Verification items for the finished model (mm, model axes). A direction names the side the tool comes from. Give positions to 0.01 mm unless a question says otherwise; leave off trailing zeros. Order: outer loops, then holes, each group sorted by start corner. A loop starts at its lowest first (then second) coordinate and runs counter-clockwise, first axis right, second up. Notation, with made-up numbers: (12, 57.25) -> (33, 57.25) arc R19 ccw to (33, 64.25) -> close; hole circle Ø10 at (88.5, -39). An arc over 180 degrees is marked (long way). Return JSON: item names as keys, results as strings. Group by question number.
(1) Release check for a two-part mould opening along Y. For faces 1 (the face through (-17.056, 75.535, 11.827)), 2 (the face through (0, 5, 28)), 3 (the face through (16.944, 75.535, 11.827)), 4 (the face through (17.06, 41.09, 31.03)) record: pulls with the +Y half, pulls with the -Y half, needs draft (parallel to the pull), parting line crosses it, or undercut.
(2) Thickness scan on line 1 along X through (y, z) = (2.75, 20); line 2 along X through (y, z) = (11, 5.5); line 3 along X through (y, z) = (3, 10). Record the ranges inside material, lowest first.
(3) Cross-section at B-B on z = 3. Enter the section's corners in (x, y).
(4) Cross-section at A-A on x = -9.5. Enter the section's corners in (y, z), then the cut area to 3 significant figures.
(5) Cross-section at D-D on x = 0. Enter the section's corners in (y, z).
(6) Depth check by flat-ended pin: pin 1 Ø2 at (x, z) = (-1.5, 28) entering from +Y; pin 2 Ø1 at (x, y) = (-15.5, 68.5) entering from +Z. Enter the tip coordinate at first touch or a pass-through.
(7) Cross-section at C-C on y = 7. Enter the section's corners in (x, z).
(8) Tool access check on faces 5 (the face through (-13, 37, 15)), 6 (the face through (16.94, 59.4, 10.81)). Record the directions out of +Z, -Z, +X, -X, +Y, -Y that give a thin tool (end or side, any length) a straight path to the whole face; none if there is none.
from build123d import *

# Parameters (mm, degrees)
DODANIE_WYCI_GNI_CIE1_DEPTH = 40
SZKIC2_R                    = 3
WYTNIJ_WYCI_GNI_CIE1_DEPTH  = 43
SZKIC3_R                    = 3
SZKIC3_R_2                  = 1.5
WYTNIJ_WYCI_GNI_CIE2_DEPTH  = 11
SZKIC4_R                    = 1.5
WYTNIJ_WYCI_GNI_CIE3_DEPTH  = 43


with BuildPart() as part:
    # Szkic1 → Dodanie-wyciągnięcie1 (new body)
    with BuildSketch(Plane.XY):
        Polygon((13, 10), (-13, 10), (-13, 80), (-21, 80), (-21, 0), (21, 0), (21, 80), (13, 80), align=None)
    extrude(amount=DODANIE_WYCI_GNI_CIE1_DEPTH)

    # Szkic2 → Wytnij-wyciągnięcie1 (cut, through all)
    with BuildSketch(Plane(origin=(21, 0, 0), x_dir=(0, 0, -1), z_dir=(1, 0, 0))):
        with BuildLine():
            Line((-40, 80), (-40, 10.986882517))
            Line((-40, 10.986882517), (-21.804909779, 72.045708909))
            ThreePointArc((-21.804909779, 72.045708909), (-17.808572792, 77.778071195), (-11.183339281, 80))
            Line((-11.183339281, 80), (-40, 80))
        make_face()
        with BuildLine():
            Line((-0.000389565, 68.866002091), (0, 10.986882517))
            Line((0, 10.986882517), (0, 80))
            Line((0, 80), (-11.085649948, 80))
            ThreePointArc((-11.085649948, 80), (-3.244243133, 76.721715095), (-0.000389565, 68.866002091))
        make_face()
        with Locations((-11.134494614, 68.866002091)):
            Circle(SZKIC2_R)
    extrude(amount=-WYTNIJ_WYCI_GNI_CIE1_DEPTH, mode=Mode.SUBTRACT)

    # Szkic3 → Wytnij-wyciągnięcie2 (cut, through all)
    with BuildSketch(Plane(origin=(0, 10, 0), x_dir=(1, 0, 0), z_dir=(0, 1, 0))):
        with Locations((0, -20)):
            Circle(SZKIC3_R)
        with Locations((0, -10.5)):
            Circle(SZKIC3_R_2)
        with Locations((9.5, -20)):
            Circle(SZKIC3_R_2)
        with Locations((0, -29.5)):
            Circle(SZKIC3_R_2)
        with Locations((-9.5, -20)):
            Circle(SZKIC3_R_2)
    extrude(amount=-WYTNIJ_WYCI_GNI_CIE2_DEPTH, mode=Mode.SUBTRACT)

    # Szkic4 → Wytnij-wyciągnięcie3 (cut, through all)
    with BuildSketch(Plane.ZY.offset(21)):
        with Locations((3.134494614, 68.866002091)):
            Circle(SZKIC4_R)
        with Locations((11.134494614, 76.866002091)):
            Circle(SZKIC4_R)
        with Locations((19.134494614, 68.866002091)):
            Circle(SZKIC4_R)
        with Locations((11.134494614, 60.866002091)):
            Circle(SZKIC4_R)
    extrude(amount=-WYTNIJ_WYCI_GNI_CIE3_DEPTH, mode=Mode.SUBTRACT)


solid = part.part
Verdict:
{
 "1": {"face 1": "undercut", "face 2": "needs draft", "face 3": "undercut", "face 4": "pulls with the +Y half"},
 "2": {"line 1": "-21 to -11, -8 to -3, 3 to 8, 11 to 21", "line 2": "-21 to -13, 13 to 21", "line 3": "-21 to -1.41, 1.41 to 21"},
 "3": {"outline": "(-21, 0) -> (21, 0) -> (21, 67.37) -> (13, 67.37) -> (13, 10) -> (-13, 10) -> (-13, 67.37) -> (-21, 67.37) -> close; (-21, 70.36) -> (-13, 70.36) -> (-13, 76.47) -> (-21, 76.47) -> close; (13, 70.36) -> (21, 70.36) -> (21, 76.47) -> (13, 76.47) -> close"},
 "4": {"outline": "(0, 0) -> (10, 0) -> (10, 18.5) -> (0, 18.5) -> close; (0, 21.5) -> (10, 21.5) -> (10, 40) -> (0, 40) -> close", "area": "370 mm²"},
 "5": {"outline": "(0, 0) -> (10, 0) -> (10, 9) -> (0, 9) -> close; (0, 12) -> (10, 12) -> (10, 17) -> (0, 17) -> close; (0, 23) -> (10, 23) -> (10, 28) -> (0, 28) -> close; (0, 31) -> (10, 31) -> (10, 40) -> (0, 40) -> close"},
 "6": {"pin 1": "y = 10", "pin 2": "z = 23.01"},
 "7": {"outline": "(-21, 0) -> (21, 0) -> (21, 40) -> (-21, 40) -> close; hole circle Ø3 at (-9.5, 20); hole circle Ø6 at (0, 20); hole circle Ø3 at (0, 10.5); hole circle Ø3 at (0, 29.5); hole circle Ø3 at (9.5, 20)"},
 "8": {"face 5": "+Z, -Z, +Y", "face 6": "+X, -X"}
}
